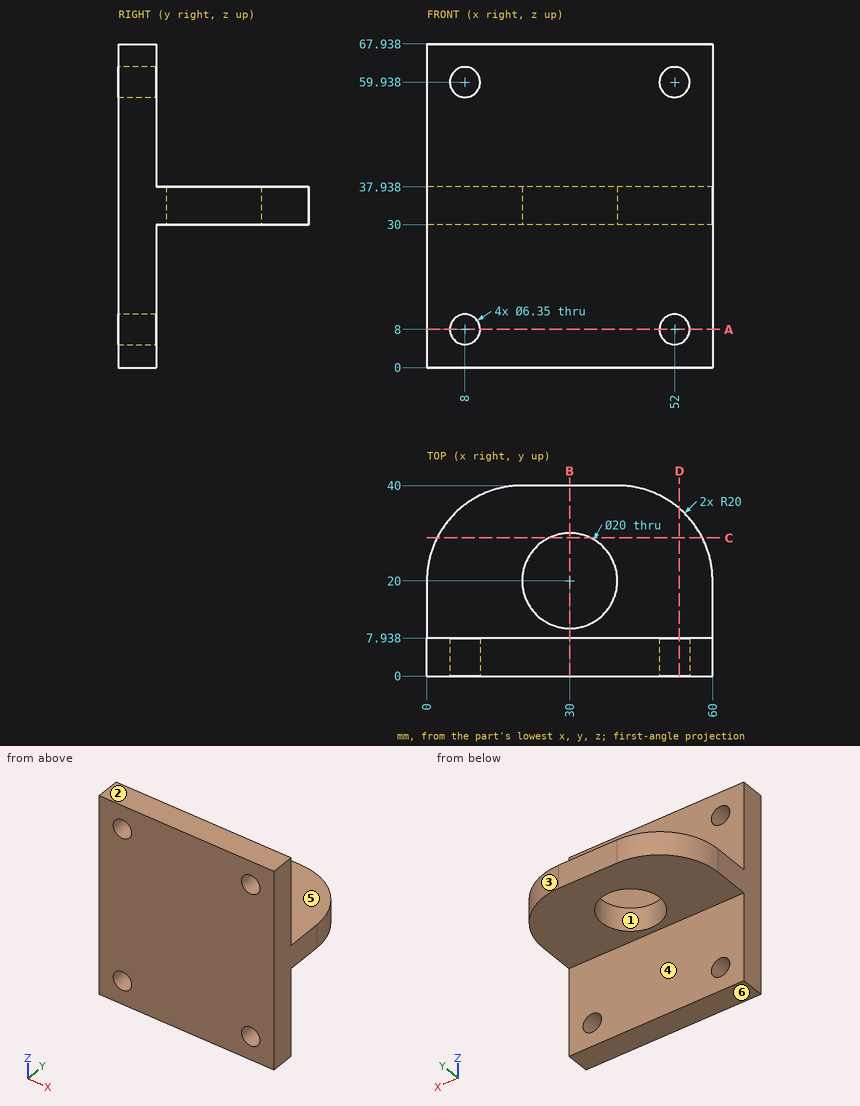
Here's the drawing with two shaded views (mm, measured from the low corner). I have some questions. A direction names the side the tool comes from. Coordinates: 2 decimals unless noted, no trailing zeros. Write each loop counter-clockwise with the first axis right and the second up, starting at its lowest first coordinate (ties: lowest second). Pieces come first, ordered by that corner, then holes. Notation, with made-up numbers: (-0.75, 22.25) -> (40.25, 22.25) arc R32 cw to (40.25, 56.25) -> close; hole circle Ø9 at (24.5, 21). An arc over 180 degrees is marked (long way). Answer as CSV lines item,"result".
1) If we mould it in two halves opening along X, with no side actions, what happens to the marked faces 1, 2 and 3? For each: +X half, -X half, draft (parallel to the pull), parting line (faces both ways), or undercut.
Check result:
face 1,"undercut"
face 2,"draft"
face 3,"+X half"
2) If we section it at B-B on x = 30: Please give me the cut outline in (y, z).
Check result:
outline,"(0, 0) -> (7.94, 0) -> (7.94, 30) -> (10, 30) -> (10, 37.94) -> (7.94, 37.94) -> (7.94, 67.94) -> (0, 67.94) -> close; (30, 30) -> (40, 30) -> (40, 37.94) -> (30, 37.94) -> close"
3) If we section it at A-A on z = 8: Please give me the cut outline in (x, y) (1 decimal).
Check result:
outline,"(0, 0) -> (4.8, 0) -> (4.8, 7.9) -> (0, 7.9) -> close; (11.2, 0) -> (48.8, 0) -> (48.8, 7.9) -> (11.2, 7.9) -> close; (55.2, 0) -> (60, 0) -> (60, 7.9) -> (55.2, 7.9) -> close"
4) Will these pins go through, and if not, where does the flat tip stop? P1, Ø8, axis at x = 52.5, y = 36, coming from the -Z side; P2, Ø8.5, axis at x = 8, z = 59.94, coming from the +Y side; P3, Ø6, axis at x = 33, y = 25.5, coming from the +Z side; P4, Ø16, axis at x = 34.5, y = 18.5, coming from the +Z side.
Check result:
P1,"z = 30"
P2,"y = 7.94"
P3,"through"
P4,"z = 37.94"
5) On a 3-axis mill with a long thin cutter (end or side, diameter ignored), from which of +Z, -Z, +X, -X, +Y, -Y can I reach the whole of each face in a straight line? I mean the marked faces 4, 5 and 6. Say none if no direction works.
Check result:
face 4,"-Z, +X, -X, +Y"
face 5,"+Z, +X, -X, +Y"
face 6,"-Z, +X, -X, +Y, -Y"
6) If we section it at C-C on y = 29: Please give me the cut outline in (x, z).
Check result:
outline,"(2.14, 30) -> (25.64, 30) -> (25.64, 37.94) -> (2.14, 37.94) -> close; (34.36, 30) -> (57.86, 30) -> (57.86, 37.94) -> (34.36, 37.94) -> close"
7) If we section it at D-D on x = 53: Count the separate pieces of the cut face and the enclosed holes in it, then the cut area to 3 significant figures.
Check result:
separate pieces,"3"
enclosed holes,"0"
area,"660 mm²"
8) If I drill on line 1 (X direction, y = 5, z = 8) (1 decimal); line 2 (Y direction, x = 30, z = 34); line 3 (X direction, y = 6, z = 10) (1 decimal), over which ranges is the centre line in solid material (lowest first)? Write a range as from..to.
Check result:
line 1,"0..4.8, 11.2..48.8, 55.2..60"
line 2,"0..10, 30..40"
line 3,"0..5.5, 10.5..49.5, 54.5..60"
